Geometry check sheet. Reference: the model listing, model coordinates, mm. A direction names the side the tool comes from. Coordinates: 2 decimals unless noted, no trailing zeros. Order: outer loops, then holes, each group sorted by start corner. A loop starts at its lowest first (then second) coordinate and runs counter-clockwise, first axis right, second up. Notation, with made-up numbers: (85.5, -29.75) - (123.5, -29.75) arc R18 ccw to (123.5, -3.75) - close; hole circle Ø9 at (-1.75, -39.75). An arc over 180 degrees is marked (long way). Return JSON: item names as keys, results as strings. Group by question number.
Item 1: Scan lines: probe 1 along Z at (x, y) = (1.65, 5.25); probe 2 along Z at (x, y) = (3.8, -5); probe 3 along Y at (x, z) = (1.2, -8). Record each from-to range of solid material in increasing order.
Item 2: Draft check along Z on faces 1 (the flat face through (2, -12.5, 0)), 2 (the cylindrical face through (1.97, -4.5, 4.55)), 3 (the flat face through (2, 0, -12.5)). Enter one of: pulls with the +Z half, pulls with the -Z half, needs draft (parallel to the pull), parting line crosses it, or undercut.
Item 3: Tool access check on faces 4 (the flat face through (1.97, 5.36, -7.62)), 5 (the flat face through (0, 0, 0)). Record the directions out of +Z, -Z, +X, -X, +Y, -Y that give a thin tool (end or side, any length) a straight path to the whole face; none if there is none.
Item 4: Section check A-A on x = 2.95. Enter the section's corners in (y, z).
from build123d import *

# Parameters (mm, degrees)
SKETCH2_W           = 25
SKETCH2_H           = 25
BOSS_EXTRUDE1_DEPTH = 4


with BuildPart() as part:
    # Sketch2 → Boss-Extrude1 (new body)
    with BuildSketch(Plane(origin=(0, 0, 0), x_dir=(0, 0, -1), z_dir=(1, 0, 0))):
        Rectangle(SKETCH2_W, SKETCH2_H)
        with BuildLine():
            Line((-4.5254834, -6.788225099), (-6.166074019, -8.428815718))
            ThreePointArc((-6.166074019, -8.428815718), (-8.428815718, -8.428815718), (-8.428815718, -6.166074019))
            Line((-8.428815718, -6.166074019), (-6.788225099, -4.5254834))
            ThreePointArc((-6.788225099, -4.5254834), (-4.5254834, -4.5254834), (-4.5254834, -6.788225099))
        make_face(mode=Mode.SUBTRACT)
        with BuildLine():
            Line((6.788225099, -4.5254834), (8.428815718, -6.166074019))
            ThreePointArc((8.428815718, -6.166074019), (8.428815718, -8.428815718), (6.166074019, -8.428815718))
            Line((6.166074019, -8.428815718), (4.5254834, -6.788225099))
            ThreePointArc((4.5254834, -6.788225099), (4.5254834, -4.5254834), (6.788225099, -4.5254834))
        make_face(mode=Mode.SUBTRACT)
        with BuildLine():
            Line((-6.788225099, 4.5254834), (-8.428815718, 6.166074019))
            ThreePointArc((-8.428815718, 6.166074019), (-8.428815718, 8.428815718), (-6.166074019, 8.428815718))
            Line((-6.166074019, 8.428815718), (-4.5254834, 6.788225099))
            ThreePointArc((-4.5254834, 6.788225099), (-4.5254834, 4.5254834), (-6.788225099, 4.5254834))
        make_face(mode=Mode.SUBTRACT)
        with BuildLine():
            Line((4.5254834, 6.788225099), (6.166074019, 8.428815718))
            ThreePointArc((6.166074019, 8.428815718), (8.428815718, 8.428815718), (8.428815718, 6.166074019))
            Line((8.428815718, 6.166074019), (6.788225099, 4.5254834))
            ThreePointArc((6.788225099, 4.5254834), (4.5254834, 4.5254834), (4.5254834, 6.788225099))
        make_face(mode=Mode.SUBTRACT)
    extrude(amount=BOSS_EXTRUDE1_DEPTH)


solid = part.part
Computed:
{
 "1": {"probe 1": "z = -12.5 to -7.51, -4.11 to 4.11, 7.51 to 12.5", "probe 2": "z = -12.5 to -7.26, -4.2 to 4.2, 7.26 to 12.5", "probe 3": "y = -12.5 to -8.73, -5.74 to 5.74, 8.73 to 12.5"},
 "2": {"face 1": "needs draft", "face 2": "undercut", "face 3": "pulls with the -Z half"},
 "3": {"face 4": "+X, -X", "face 5": "+Z, -Z, -X, +Y, -Y"},
 "4": {"outline": "(-12.5, -12.5) - (12.5, -12.5) - (12.5, 12.5) - (-12.5, 12.5) - close; hole (-8.43, -6.17) arc R1.6 ccw to (-6.17, -8.43) - (-4.53, -6.79) arc R1.6 ccw to (-6.79, -4.53) - close; hole (-8.43, 6.17) - (-6.79, 4.53) arc R1.6 ccw to (-4.53, 6.79) - (-6.17, 8.43) arc R1.6 ccw to start; hole (4.53, -6.79) - (6.17, -8.43) arc R1.6 ccw to (8.43, -6.17) - (6.79, -4.53) arc R1.6 ccw to start; hole (4.53, 6.79) arc R1.6 ccw to (6.79, 4.53) - (8.43, 6.17) arc R1.6 ccw to (6.17, 8.43) - close"}
}
